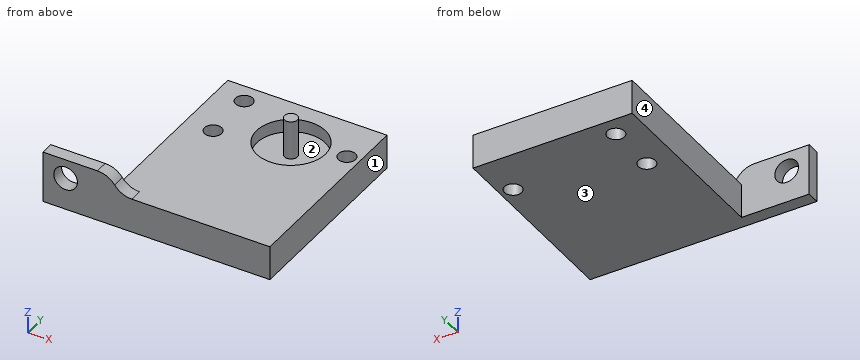
```python
from build123d import *

# Parameters (mm, degrees)
ESQUISSE1_W             = 37
ESQUISSE1_H             = 42.25
ESQUISSE1_R             = 6
BOSS_EXTRU_1_DEPTH      = 12
ESQUISSE2_R             = 6
ESQUISSE2_R_2           = 1.5
ENL_V_MAT_EXTRU_1_DEPTH = 3
ESQUISSE3_W             = 37
ESQUISSE3_H             = 12
ESQUISSE3_W_2           = 15.75
ESQUISSE3_R             = 2.75
BOSS_EXTRU_2_DEPTH      = 3
ESQUISSE4_W             = 37
ESQUISSE4_H             = 45.25
ESQUISSE4_R             = 8
ENL_V_MAT_EXTRU_2_DEPTH = 4
ESQUISSE4_3_R           = 8
ESQUISSE4_3_R_2         = 6
ESQUISSE4_3_R_3         = 1.5
ENL_V_MAT_EXTRU_4_DEPTH = 7
CONG_2_R                = 5
CONG_3_R                = 5
ESQUISSE5_R             = 2
ENL_V_MAT_EXTRU_5_DEPTH = 43.650652105
BOSS_EXTRU_3_START      = 2
ESQUISSE2_2_R           = 1.5
BOSS_EXTRU_3_DEPTH      = 2


with BuildPart() as part:
    # Esquisse1 → Boss.-Extru.1 (new body)
    # profile 1 of 2: a face of its own
    with BuildSketch(Plane.XY):
        Rectangle(ESQUISSE1_W, ESQUISSE1_H)
        with Locations((3.4, 9.125)):
            Circle(ESQUISSE1_R, mode=Mode.SUBTRACT)
    # profile 2 of 2: a face of its own
    with BuildSketch(Plane.XY):
        with Locations((3.4, 9.125)):
            Circle(ESQUISSE1_R)
    extrude(amount=BOSS_EXTRU_1_DEPTH)

    # Esquisse2 → Enlèv. mat.-Extru.1 (cut)
    with BuildSketch(Plane.XY.offset(12)):
        with Locations((3.4, 9.125)):
            Circle(ESQUISSE2_R)
        with Locations((3.4, 9.125)):
            Circle(ESQUISSE2_R_2, mode=Mode.SUBTRACT)
    extrude(amount=-ENL_V_MAT_EXTRU_1_DEPTH, mode=Mode.SUBTRACT)

    # Esquisse3 → Boss.-Extru.2 (add)
    # profile 1 of 2: a face of its own
    with BuildSketch(Plane.XZ.offset(21.125)):
        with Locations((0, 6)):
            Rectangle(ESQUISSE3_W, ESQUISSE3_H)
    # profile 2 of 2: a face of its own
    with BuildSketch(Plane.XZ.offset(21.125)):
        with Locations((-26.375, 6)):
            Rectangle(ESQUISSE3_W_2, ESQUISSE3_H)
        with Locations((-29, 7.5)):
            Circle(ESQUISSE3_R, mode=Mode.SUBTRACT)
    extrude(amount=BOSS_EXTRU_2_DEPTH)

    # Esquisse4 → Enlèv. mat.-Extru.2 (cut)
    with BuildSketch(Plane.XY.offset(12)):
        with Locations((0, -1.5)):
            Rectangle(ESQUISSE4_W, ESQUISSE4_H)
        with Locations((3.4, 9.125)):
            Circle(ESQUISSE4_R, mode=Mode.SUBTRACT)
    extrude(amount=-ENL_V_MAT_EXTRU_2_DEPTH, mode=Mode.SUBTRACT)

    # Esquisse4<3> → Enlèv. mat.-Extru.4 (cut)
    # profile 1 of 2: a face of its own
    with BuildSketch(Plane.XY.offset(12)):
        with Locations((3.4, 9.125)):
            Circle(ESQUISSE4_3_R)
        with Locations((3.4, 9.125)):
            Circle(ESQUISSE4_3_R_2, mode=Mode.SUBTRACT)
    # profile 2 of 2: a face of its own
    with BuildSketch(Plane.XY.offset(12)):
        with Locations((3.4, 9.125)):
            Circle(ESQUISSE4_3_R_2)
        with Locations((3.4, 9.125)):
            Circle(ESQUISSE4_3_R_3, mode=Mode.SUBTRACT)
    extrude(amount=-ENL_V_MAT_EXTRU_4_DEPTH, mode=Mode.SUBTRACT)

    # Congé2
    # the kernel refuses this fillet: 5 mm, written as the material it adds along each edge
    with BuildSketch(Plane(origin=(-18.5, -24.125, 8), x_dir=(1.5667467323505199e-12, 0, 1.0), z_dir=(0, 1, 0))) as cong_2_piece_1:
        with BuildLine():
            CenterArc((5, 4.898979486), CONG_2_R, 180, 78.463040967)
            Line((0, 4.898979486), (0, 0))
            Line((0, 0), (4, 0))
        make_face()
    extrude(amount=3)

    # Congé3
    cong_3_edges = [part.edges().sort_by_distance(p)[0] for p in [
        (-18.5, -22.625, 12),
    ]]
    fillet(cong_3_edges, radius=CONG_3_R)

    # Esquisse5 → Enlèv. mat.-Extru.5 (cut, through all)
    with BuildSketch(Plane.XY.offset(8)):
        with Locations((-12, 16.625)):
            Circle(ESQUISSE5_R)
        with Locations((-12, 4.625)):
            Circle(ESQUISSE5_R)
        with Locations((15.5, 10.625)):
            Circle(ESQUISSE5_R)
    extrude(amount=-ENL_V_MAT_EXTRU_5_DEPTH, mode=Mode.SUBTRACT)

    # Esquisse2<2> → Boss.-Extru.3 (add)
    with BuildSketch(Plane.XY.offset(12).offset(BOSS_EXTRU_3_START)):
        with Locations((3.4, 9.125)):
            Circle(ESQUISSE2_2_R)
    extrude(amount=-BOSS_EXTRU_3_DEPTH)


solid = part.part
```
Check sheet for the modelled part. Datum: model origin and axes. Units: mm. Face numbers are marked on the shaded views. Round coordinates to 2 decimals unless told otherwise and drop trailing zeros. Order: outer loops, then holes, each group sorted by start corner. A loop starts at its lowest first (then second) coordinate and runs counter-clockwise, first axis right, second up. Notation, with made-up numbers: (61.5, 49) - (89.5, 49) arc R19 ccw to (89.5, 72) - close; hole circle Ø1 at (0.5, -10). An arc over 180 degrees is marked (long way). Answer as CSV lines item,"result". Start each with the question number.
1) Section check D-D (x = 3.4). Record the cut outline in (y, z) (3 decimals), then the cut area to 3 significant figures.
2) Depth check by flat-ended pin: pin 1 (9.5 mm diameter, centred on x = 3.4, y = 9.125, fed in from -Z); pin 2 (0.9 mm diameter, centred on x = -26.5, y = -22, fed in from +Z); pin 3 (3 mm diameter, centred on y = -3, z = 8.5, fed in from -X); pin 4 (6 mm diameter, centred on x = -15.5, y = -5, fed in from +Z). Enter the tip coordinate at first touch or a pass-through.
3) Section check B-B (y = 15.5). Record the cut outline in (x, z), then the cut area to 3 significant figures.
4) Section check C-C (z = 6.5). Record the cut outline in (x, y) (3 decimals).
5) Scan lines: probe 1 along Y at (x, z) = (-12, 2.5) (3 decimals); probe 2 along Z at (x, y) = (-29, -22); probe 3 along X at (y, z) = (-15, 2). Record each from-to range of solid material in increasing order.
6) Draft check along X on the marked faces 1, 2, 3 and 4. Enter one of: +X half, -X half, draft (parallel to the pull), parting line (faces both ways), or undercut.
7) Section check A-A (x = -29). Record the cut outline in (y, z) (3 decimals).
Determined:
1,outline,"(-24.125, 0) - (21.125, 0) - (21.125, 8) - (17.125, 8) - (17.125, 5) - (10.625, 5) - (10.625, 14) - (7.625, 14) - (7.625, 5) - (1.125, 5) - (1.125, 8) - (-24.125, 8) - close"
1,area,"341 mm^2"
2,pin 1,"z = 0"
2,pin 2,"z = 12"
2,pin 3,"x = -18.5"
2,pin 4,"z = 8"
3,outline,"(-18.5, 0) - (-13.65, 0) - (-13.65, 8) - (-18.5, 8) - close; (-10.35, 0) - (18.5, 0) - (18.5, 8) - (8.23, 8) - (8.23, 5) - (-1.43, 5) - (-1.43, 8) - (-10.35, 8) - close"
3,area,"241 mm^2"
4,outline,"(-34.25, -24.125) - (-31.562, -24.125) - (-31.562, -21.125) - (-34.25, -21.125) - close; (-26.438, -24.125) - (18.5, -24.125) - (18.5, 21.125) - (-18.5, 21.125) - (-18.5, -21.125) - (-26.438, -21.125) - close; circle Ø3 at (3.4, 9.125); hole circle Ø4 at (-12, 4.625); hole circle Ø4 at (-12, 16.625); hole circle Ø16 at (3.4, 9.125); hole circle Ø4 at (15.5, 10.625)"
5,probe 1,"-24.125 to 2.625, 6.625 to 14.625, 18.625 to 21.125"
5,probe 2,"0 to 4.75, 10.25 to 12"
5,probe 3,"-18.5 to 18.5"
6,face 1,"+X half"
6,face 2,"undercut"
6,face 3,"draft"
6,face 4,"-X half"
7,outline,"(-24.125, 0) - (-21.125, 0) - (-21.125, 4.75) - (-24.125, 4.75) - close; (-24.125, 10.25) - (-21.125, 10.25) - (-21.125, 12) - (-24.125, 12) - close"
